Can you work these out from the model? Positions are in its coordinate system, mm. Face numbers are marked on the shaded views. A direction names the side the tool comes from. Give positions to 0.01 mm unless a question says otherwise; leave off trailing zeros. Order: outer loops, then holes, each group sorted by start corner. A loop starts at its lowest first (then second) coordinate and runs counter-clockwise, first axis right, second up. Notation, with made-up numbers: (6.5, -37.75) - (30.5, -37.75) arc R14 cw to (30.5, -10.75) - close; hole circle Ø5 at (2, 59). An arc over 180 degrees is marked (long way). Return JSON: item names as keys, results as strings.
```python
from build123d import *

# Parameters (mm, degrees)
F0_R      = 15
F1_DEPTH  = 5
F2_R      = 15
F3_DEPTH  = 5
F4_R      = 5
F6_R      = 20
F7_DEPTH  = 5
F8_R      = 20
F9_DEPTH  = 5
F10_R     = 3.1
F11_DEPTH = 25
F10_R_2   = 5
F12_DEPTH = 3
F13_R     = 5
F13_R_2   = 3.1
F14_DEPTH = 3


with BuildPart() as f1:
    # F0 (on Front) → F1 (new body)
    with BuildSketch(Plane.XZ):
        Circle(F0_R)
    extrude(amount=F1_DEPTH)

    # F2 (on face) → F3 (join)
    with BuildSketch(Plane(origin=(0, 0, 0), x_dir=(-1, 0, 0), z_dir=(0, 1, 0))):
        Circle(F2_R)
    extrude(amount=F3_DEPTH)

    # F5: sweep along a path in F2
    with BuildLine(Plane(origin=(0, 0, 0), x_dir=(-1, 0, 0), z_dir=(0, 1, 0))) as f5_path:
        CenterArc((0, 0), 15, 0, 360)
    # F4 (on Right) → F5 (sweep, cut)
    with BuildSketch(Plane.YZ):
        with Locations((0, -15)):
            Circle(F4_R)
    sweep(path=f5_path.line, mode=Mode.SUBTRACT)

    # F6 (on face) → F7 (join)
    with BuildSketch(Plane.XZ.offset(5)):
        Circle(F6_R)
    extrude(amount=F7_DEPTH)

    # F8 (on face) → F9 (join)
    with BuildSketch(Plane(origin=(0, 5, 0), x_dir=(-1, 0, 0), z_dir=(0, 1, 0))):
        Circle(F8_R)
    extrude(amount=F9_DEPTH)

    # F10 (on face) → F11 (cut)
    with BuildSketch(Plane.XZ.offset(10)):
        Circle(F10_R)
    extrude(amount=-F11_DEPTH, mode=Mode.SUBTRACT)

    # F10 (on face) → F12 (cut)
    with BuildSketch(Plane.XZ.offset(10)):
        Circle(F10_R_2)
        Circle(F10_R, mode=Mode.SUBTRACT)
    extrude(amount=-F12_DEPTH, mode=Mode.SUBTRACT)

    # F13 (on face) → F14 (cut)
    with BuildSketch(Plane(origin=(0, 10, 0), x_dir=(-1, 0, 0), z_dir=(0, 1, 0))):
        Circle(F13_R)
        Circle(F13_R_2, mode=Mode.SUBTRACT)
    extrude(amount=-F14_DEPTH, mode=Mode.SUBTRACT)


solid = f1.part
```
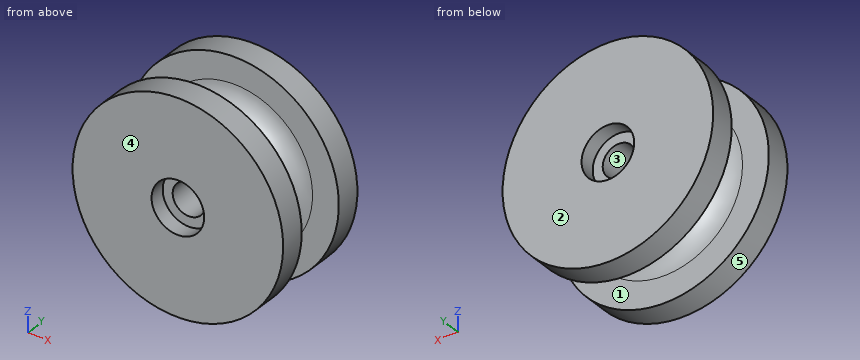
1. For pin 1 Ø2 at (y, z) = (-5, 5.5) entering from +X; pin 2 Ø3 at (x, z) = (2, -1) entering from +Y; pin 3 Ø3 at (x, y) = (15.5, -4) entering from +Z, each with a flat end and sliding along its axis, tell me the tip position at first contact or that it passes through.
Checks:
{"pin 1": "x = 19.49", "pin 2": "y = 7", "pin 3": "z = 13.9"}
2. Suppose I cut it at A-A (z = 0). List the corners of the cut face in (x, y) for me.
Checks:
{"outline": "(-20, -10) - (-5, -10) - (-5, -7) - (-3.1, -7) - (-3.1, 7) - (-5, 7) - (-5, 10) - (-20, 10) - (-20, 5) - (-15, 5) arc R5 cw to (-15, -5) - (-20, -5) - close; (3.1, -7) - (5, -7) - (5, -10) - (20, -10) - (20, -5) - (15, -5) arc R5 cw to (15, 5) - (20, 5) - (20, 10) - (5, 10) - (5, 7) - (3.1, 7) - close"}
3. Suppose I cut it at B-B (x = 0). List the corners of the cut face in (y, z) for me, plus the area to 3 significant figures.
Checks:
{"outline": "(-10, -20) - (-5, -20) - (-5, -15) arc R5 cw to (5, -15) - (5, -20) - (10, -20) - (10, -5) - (7, -5) - (7, -3.1) - (-7, -3.1) - (-7, -5) - (-10, -5) - close; (-10, 5) - (-7, 5) - (-7, 3.1) - (7, 3.1) - (7, 5) - (10, 5) - (10, 20) - (5, 20) - (5, 15) arc R5 cw to (-5, 15) - (-5, 20) - (-10, 20) - close", "area": "475 mm^2"}
4. If I drill on L1, parallel to Y at x = 14, z = -8.5; L2, parallel to Z at x = 0, y = -8.75; L3, parallel to Y at x = -6, z = 11.5, over which ranges is the centre line in solid material (lowest first)? Write a range as [from, to].
Checks:
{"L1": "[-10, -5], [5, 10]", "L2": "[-20, -5], [5, 20]", "L3": "[-10, -4.57], [4.57, 10]"}
5. On a 3-axis mill with a long thin cutter (end or side, diameter ignored), from which of +Z, -Z, +X, -X, +Y, -Y can I reach the whole of each face in a straight line? I mean the marked faces 1 and 2. Say none if no direction works.
Checks:
{"face 1": "none", "face 2": "+Z, -Z, +X, -X, +Y"}
6. Suppose I cut it at C-C (y = -6). List the corners of the cut face in (x, z) for me, plus the area to 3 significant figures.
Checks:
{"outline": "circle Ø40 at (0, 0); hole circle Ø6.2 at (0, 0)", "area": "1,230 mm^2"}
7. Thinking about a two-plate mould opening in Z: for the marked faces 3, 4 and 5, which applies, +Z half, -Z half, draft (parallel to the pull), parting line (faces both ways), or undercut?
Checks:
{"face 3": "undercut", "face 4": "draft", "face 5": "parting line"}
8. Suppose I cut it at D-D (z = 17.5). List the corners of the cut face in (x, y) for me.
Checks:
{"outline": "(-9.68, -10) - (9.68, -10) - (9.68, -5) - (-9.68, -5) - close; (-9.68, 5) - (9.68, 5) - (9.68, 10) - (-9.68, 10) - close"}
